from build123d import *

# Parameters (mm, degrees)
SKETCH1_R           = 14
BOSS_EXTRUDE1_DEPTH = 6
BOSS_EXTRUDE1_TAPER = 66
BOSS_EXTRUDE2_DEPTH = 145
SKETCH3_R           = 16
BOSS_EXTRUDE3_DEPTH = 3


with BuildPart() as part:
    # Sketch1 → Boss-Extrude1 (new body)
    with BuildSketch(Plane(origin=(0, 0, 0), x_dir=(0, 0, -1), z_dir=(1, 0, 0))):
        Circle(SKETCH1_R)
    extrude(amount=BOSS_EXTRUDE1_DEPTH, taper=BOSS_EXTRUDE1_TAPER)

    # Sketch2 → Boss-Extrude2 (add)
    with BuildSketch(Plane.ZY):
        Polygon((1.5, -1.5), (1.5, -13.919410907), (-1.5, -13.919410907), (-1.5, -1.5), (-13.919410907, -1.5), (-13.919410907, 1.5), (-1.5, 1.5), (-1.5, 13.919410907), (1.5, 13.919410907), (1.5, 1.5), (13.919410907, 1.5), (13.919410907, -1.5), align=None)
    extrude(amount=BOSS_EXTRUDE2_DEPTH)

    # Sketch3 → Boss-Extrude3 (add)
    with BuildSketch(Plane.ZY.offset(145)):
        Circle(SKETCH3_R)
    extrude(amount=BOSS_EXTRUDE3_DEPTH)


solid = part.part
Can you work these out from the model? Positions are in its coordinate system, mm. A direction names the side the tool comes from. Coordinates: 2 decimals unless noted, no trailing zeros. Write each loop counter-clockwise with the first axis right and the second up, starting at its lowest first coordinate (ties: lowest second). Pieces come first, ordered by that corner, then holes. Notation, with made-up numbers: (-31, -35) -> (-21, -35) arc R9 cw to (-21, -20) -> close; hole circle Ø10 at (65, 40). An arc over 180 degrees is marked (long way). Write each question's results on one line, items separated by ' | '. Start each with the question number.
Item 1: Please list where these lines run through material, in increasing order: probe 1 along X at (y, z) = (2.5, 12.5); probe 2 along X at (y, z) = (-6.5, -12.5); probe 3 along Z at (x, y) = (-4, 5).
Item 2: Thinking about a two-plate mould opening in X: for faces 1 (the flat face through (-148, 0, 0)), 2 (the flat face through (-71, 8, -1.5)), which applies, released by +X, released by -X, zero draft, split by the parting line, or undercut?
Item 3: If we section it at A-A, the plane x = -115: Write out the boundary of the cut face in (y, z), and give its area (3 significant figures).
Item 4: On a 3-axis mill with a long thin cutter (end or side, diameter ignored), from which of +Z, -Z, +X, -X, +Y, -Y can I reach the whole of each face in a straight line? I mean faces 3 (the flat face through (-71, -1.5, -8)), 4 (the flat face through (0, -6, 6)). Say none if no direction works.
Item 5: I'm going to push flat-ended pins straight in: P1, Ø5, axis at x = -78, y = -10.5, coming from the -Z side; P2, Ø3.5, axis at x = -98, z = -0.5, coming from the -Y side; P3, Ø1.5, axis at x = -52.5, y = 0.5, coming from the +Z side. Where does each tip first touch, or does it pass through?
Answer block:
1) probe 1: -148 to -145, 0 to 0.56 | probe 2: -148 to -145 | probe 3: -1.5 to 1.5
2) face 1: released by -X | face 2: undercut
3) outline: (-13.92, -1.5) -> (-1.5, -1.5) -> (-1.5, -13.92) -> (1.5, -13.92) -> (1.5, -1.5) -> (13.92, -1.5) -> (13.92, 1.5) -> (1.5, 1.5) -> (1.5, 13.92) -> (-1.5, 13.92) -> (-1.5, 1.5) -> (-13.92, 1.5) -> close | area: 158 mm²
4) face 3: -Z, -Y | face 4: +Z, -Y
5) P1: z = -1.5 | P2: y = -13.92 | P3: z = 13.92
